Input: part model. Units: mm. Frame: model coordinates. Face numbers are marked on the shaded views. Coordinates: 2 decimals unless noted, no trailing zeros. Write each loop counter-clockwise with the first axis right and the second up, starting at its lowest first coordinate (ties: lowest second). Pieces come first, ordered by that corner, then holes. Notation, with made-up numbers: M -12,72.5 L 16,72.5 A26 cw 16,98.5 Z; hole C 41.25,20 d10. An arc over 180 degrees is marked long. Use one line per item in the form item = value.
from build123d import *

# Parameters (mm, degrees)
SKETCH1_W             = 30
SKETCH1_H             = 30
BOSS_EXTRUDE1_DEPTH   = 3
M4X0_7_TAPPED_HOLE1_D = 3.3
CHAMFER2_SIZE         = 3


with BuildPart() as part:
    # Sketch1 → Boss-Extrude1 (new body)
    with BuildSketch(Plane(origin=(0, 0, 0), x_dir=(1, 0, 0), z_dir=(0, 1, 0))):
        Rectangle(SKETCH1_W, SKETCH1_H)
    extrude(amount=BOSS_EXTRUDE1_DEPTH)

    # M4x0.7 Tapped Hole1 (through all)
    with Locations(Plane(origin=(0, 3, 0), x_dir=(1, 0, 0), z_dir=(0, 1, 0))):
        with Locations((-10, -10), (-10, 10), (10, 10), (10, -10)):
            Hole(M4X0_7_TAPPED_HOLE1_D / 2)

    # Chamfer2
    chamfer2_edges = [part.edges().sort_by_distance(p)[0] for p in [
        (0, 3, 15),
    ]]
    chamfer(chamfer2_edges, length=CHAMFER2_SIZE - 0.0001)  # a hair under: the kernel refuses the full size


solid = part.part
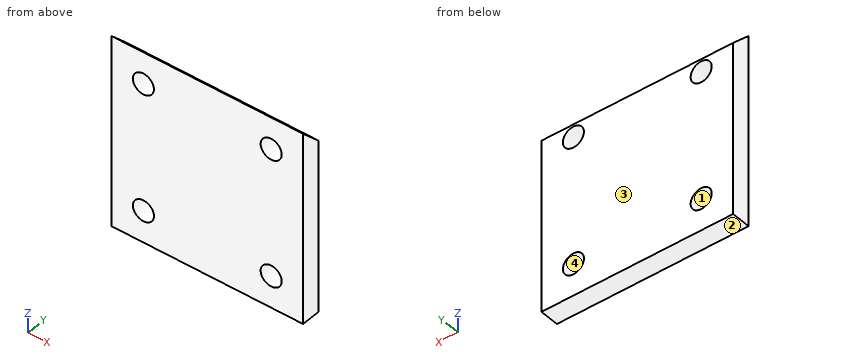
(1) Section query C-C on y = 1.15. Return the cut outline in (x, z).
Computed:
outline = M -15,-15 L 15,-15 L 15,13.85 L -15,13.85 Z; hole C -10,-10 d3.3; hole C -10,10 d3.3; hole C 10,-10 d3.3; hole C 10,10 d3.3
(2) Section query A-A on z = 10. Return the cut outline in (x, y), plus the area to 3 significant figures.
Computed:
outline = M -15,0 L -11.65,0 L -11.65,3 L -15,3 Z; M -8.35,0 L 8.35,0 L 8.35,3 L -8.35,3 Z; M 11.65,0 L 15,0 L 15,3 L 11.65,3 Z
area = 70.2 mm^2
(3) Pull-direction query (Z, two-part tool) for the marked faces 1, 2, 3 and 4; classes: pulls with the +Z half, pulls with the -Z half, needs draft (parallel to the pull), parting line crosses it, or undercut.
Computed:
face_1 = undercut
face_2 = pulls with the -Z half
face_3 = needs draft
face_4 = undercut
(4) Section query B-B on x = -10. State how many separate pieces and enclosed holes the cut face has, plus the area to 3 significant figures.
Computed:
separate_pieces = 3
enclosed_holes = 0
area = 65.7 mm^2
(5) First-contact query: pin 1 Ø12 at (x, z) = (-11.5, 6) entering from -Y; pin 2 Ø1 at (x, y) = (-2.5, 2) entering from +Z. Flat tips, straight axial feed; report the tip coordinate or a pass-through.
Computed:
pin_1 = 0
pin_2 = 13.5
(6) Line query: probe 1 along X at (y, z) = (1.4, 10); probe 2 along Z at (x, y) = (10, 0.7); probe 3 along Z at (x, y) = (-10, 1.2). Output: solid intervals per line, ascending.
Computed:
probe_1 = -15 to -11.65, -8.35 to 8.35, 11.65 to 15
probe_2 = -15 to -11.65, -8.35 to 8.35, 11.65 to 14.3
probe_3 = -15 to -11.65, -8.35 to 8.35, 11.65 to 13.8
